```python
from build123d import *

# Parameters (mm, degrees)
SKETCH_1_R          = 10
EXTRUDE_1_DEPTH     = 2
CUT_EXTRUDE_1_REACH = 16.283
SKETCH_2_R          = 1.5
SKETCH_3_R          = 4.75
SKETCH_3_R_2        = 3
EXTRUDE_2_DEPTH     = 3.5


with BuildPart() as part:
    # 草图1 → 凸台-拉伸1 (new body)
    with BuildSketch(Plane.XY):
        Circle(SKETCH_1_R)
    extrude(amount=-EXTRUDE_1_DEPTH)

    # 草图2 → 切除-拉伸1 (cut, up to next)
    with BuildSketch(Plane.XY, mode=Mode.PRIVATE) as cut_extrude_1_sk1:
        Circle(SKETCH_2_R)
    cut_extrude_1_tool1 = extrude(cut_extrude_1_sk1.sketch, amount=-CUT_EXTRUDE_1_REACH, mode=Mode.PRIVATE) & part.part
    # 草图2 → 切除-拉伸1 (cut, up to next)
    with BuildSketch(Plane.XY, mode=Mode.PRIVATE) as cut_extrude_1_sk2:
        with Locations((-7.1, 0)):
            Circle(SKETCH_2_R)
    cut_extrude_1_tool2 = extrude(cut_extrude_1_sk2.sketch, amount=-CUT_EXTRUDE_1_REACH, mode=Mode.PRIVATE) & part.part
    # 草图2 → 切除-拉伸1 (cut, up to next)
    with BuildSketch(Plane.XY, mode=Mode.PRIVATE) as cut_extrude_1_sk3:
        with Locations((0, 7.1)):
            Circle(SKETCH_2_R)
    cut_extrude_1_tool3 = extrude(cut_extrude_1_sk3.sketch, amount=-CUT_EXTRUDE_1_REACH, mode=Mode.PRIVATE) & part.part
    # 草图2 → 切除-拉伸1 (cut, up to next)
    with BuildSketch(Plane.XY, mode=Mode.PRIVATE) as cut_extrude_1_sk4:
        with Locations((7.1, 0)):
            Circle(SKETCH_2_R)
    cut_extrude_1_tool4 = extrude(cut_extrude_1_sk4.sketch, amount=-CUT_EXTRUDE_1_REACH, mode=Mode.PRIVATE) & part.part
    # 草图2 → 切除-拉伸1 (cut, up to next)
    with BuildSketch(Plane.XY, mode=Mode.PRIVATE) as cut_extrude_1_sk5:
        with Locations((0, -7.1)):
            Circle(SKETCH_2_R)
    cut_extrude_1_tool5 = extrude(cut_extrude_1_sk5.sketch, amount=-CUT_EXTRUDE_1_REACH, mode=Mode.PRIVATE) & part.part
    add(cut_extrude_1_tool1.solids().sort_by_distance((0, 0, 0))[0], mode=Mode.SUBTRACT)
    add(cut_extrude_1_tool2.solids().sort_by_distance((-7.1, 0, 0))[0], mode=Mode.SUBTRACT)
    add(cut_extrude_1_tool3.solids().sort_by_distance((0, 7.1, 0))[0], mode=Mode.SUBTRACT)
    add(cut_extrude_1_tool4.solids().sort_by_distance((7.1, 0, 0))[0], mode=Mode.SUBTRACT)
    add(cut_extrude_1_tool5.solids().sort_by_distance((0, -7.1, 0))[0], mode=Mode.SUBTRACT)

    # 草图3 → 凸台-拉伸2 (add)
    with BuildSketch(Plane(origin=(0, 0, -2), x_dir=(-1, 0, 0), z_dir=(0, 0, -1))):
        with Locations(Location((0, 0, 0), (0, 0, 180))):
            Circle(SKETCH_3_R)
        Circle(SKETCH_3_R_2, mode=Mode.SUBTRACT)
    extrude(amount=EXTRUDE_2_DEPTH)


solid = part.part
```
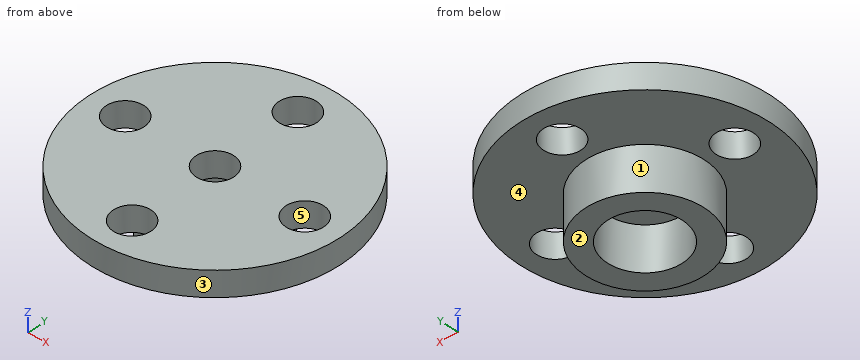
Verification items for the finished model (mm, model axes). Face numbers are marked on the shaded views. A direction names the side the tool comes from. Coordinates: 2 decimals unless noted, no trailing zeros. Loops run counter-clockwise (first coordinate to the right, second up) from the corner with the lowest first, then second, coordinate; pieces in that order, holes last. Notation, with made-up numbers: (-30.5, -6) -> (-1.5, -6) arc R8 cw to (-1.5, 4) -> close; hole circle Ø7 at (30, 39). An arc over 180 degrees is marked (long way). Answer in a Markdown table with one row per item. Add a question column.
1. Access from +Z, -Z, +X, -X, +Y, -Y to the whole of each face (thin tool, end or side, straight path). Record for the marked faces 1 and 2.
2. Section check D-D, the plane z = -0.85. Enter the section's corners in (x, y).
3. Draft check along X on the marked faces 3, 4 and 5. Enter one of: +X half, -X half, draft (parallel to the pull), parting line (faces both ways), or undercut.
4. Section check B-B, the plane x = 0. Enter the section's corners in (y, z), then the cut area to 4 significant figures.
5. Section check A-A, the plane x = 8. Enter the section's corners in (y, z), then the cut area to 3 significant figures.
6. Material ranges on probe 1 along Y at (x, z) = (0, -0.45); probe 2 along Y at (x, z) = (0, -3.65); probe 3 along Z at (x, y) = (-6.25, 4), recorded low to high. Write a range as [from, to].
7. Depth check by flat-ended pin: P1, Ø1, axis at x = 7.5, z = -2, coming from the +Y side; P2, Ø1, axis at x = -5, z = -2, coming from the +Y side. Enter the tip coordinate at first touch or a pass-through.
Derived:
| question | item | result |
|---|---|---|
| 1 | face 1 | -Z |
| 1 | face 2 | -Z, +X, -X, +Y, -Y |
| 2 | outline | circle Ø20 at (0, 0); hole circle Ø3 at (-7.1, 0); hole circle Ø3 at (0, -7.1); hole circle Ø3 at (0, 0); hole circle Ø3 at (0, 7.1); hole circle Ø3 at (7.1, 0) |
| 3 | face 3 | parting line |
| 3 | face 4 | draft |
| 3 | face 5 | undercut |
| 4 | outline | (-10, -2) -> (-8.6, -2) -> (-8.6, 0) -> (-10, 0) -> close; (-5.6, -2) -> (-4.75, -2) -> (-4.75, -5.5) -> (-3, -5.5) -> (-3, -2) -> (-1.5, -2) -> (-1.5, 0) -> (-5.6, 0) -> close; (1.5, -2) -> (3, -2) -> (3, -5.5) -> (4.75, -5.5) -> (4.75, -2) -> (5.6, -2) -> (5.6, 0) -> (1.5, 0) -> close; (8.6, -2) -> (10, -2) -> (10, 0) -> (8.6, 0) -> close |
| 4 | area | 34.25 mm² |
| 5 | outline | (-6, -2) -> (-1.2, -2) -> (-1.2, 0) -> (-6, 0) -> close; (1.2, -2) -> (6, -2) -> (6, 0) -> (1.2, 0) -> close |
| 5 | area | 19.2 mm² |
| 6 | probe 1 | y = [-10, -8.6], [-5.6, -1.5], [1.5, 5.6], [8.6, 10] |
| 6 | probe 2 | y = [-4.75, -3], [3, 4.75] |
| 6 | probe 3 | z = [-2, 0] |
| 7 | P1 | stops at y = 7.14 |
| 7 | P2 | stops at y = 8.93 |
